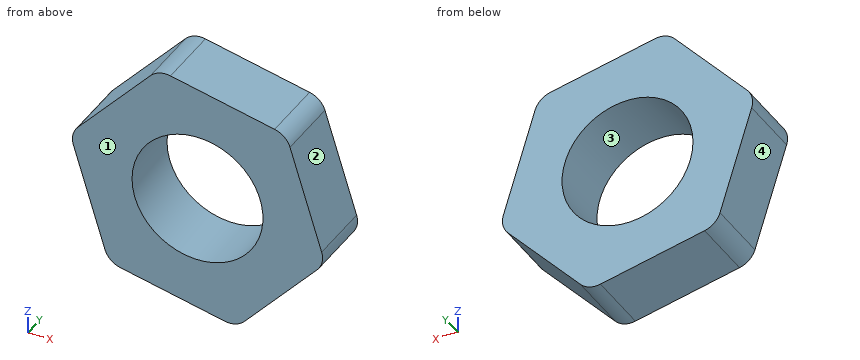
```python
from build123d import *

# Parameters (mm, degrees)
F1_DEPTH = 1.190625
F2_R     = 2.38125
F3_DEPTH = 2.38125
F4_R     = 0.762


with BuildPart() as f1:
    # F0 (on Front) → F1 (new body, symmetric)
    with BuildSketch(Plane.XZ):
        Polygon((-1.4126416008, 4.548169957), (-4.6451515239, 1.0507014657), (-3.2325099231, -3.4974684913), (1.4126416008, -4.548169957), (4.6451515239, -1.0507014657), (3.2325099231, 3.4974684913), align=None)
    extrude(amount=F1_DEPTH, both=True)

    # F2 (on face) → F3 (cut)
    with BuildSketch(Plane(origin=(0, 1.190625, 0), x_dir=(-1, 0, 0), z_dir=(0, 1, 0))):
        Circle(F2_R)
    extrude(amount=-F3_DEPTH, mode=Mode.SUBTRACT)

    # F4
    f4_edges = [f1.edges().sort_by_distance(p)[0] for p in [
        (-1.412642, 0, 4.54817),
        (3.23251, 0, 3.497468),
        (4.645152, 0, -1.050701),
        (1.412642, 0, -4.54817),
        (-3.23251, 0, -3.497468),
        (-4.645152, 0, 1.050701),
    ]]
    fillet(f4_edges, radius=F4_R)


solid = f1.part
```
CAD build for the part. Positions are in the model's coordinates, mm. Face numbers are marked on the shaded views. Round coordinates to 2 decimals unless told otherwise and drop trailing zeros. Write each loop counter-clockwise with the first axis right and the second up, starting at its lowest first coordinate (ties: lowest second). Pieces come first, ordered by that corner, then holes. Notation, with made-up numbers: (-10.5, 79) -> (12.5, 79) arc R5 ccw to (12.5, 83) -> close; hole circle Ø3 at (-20, 40.5). An arc over 180 degrees is marked (long way). Answer in a Markdown table with one row per item. Add a question column.
Item 1: Saw through at A-A, the plane y = 0.2. Write the cut outline in (x, z), then the cut area to 3 significant figures.
Item 2: Drill centre lines: line 1 (Z direction, x = 0, y = -0.25); line 2 (Z direction, x = 1.5, y = 0.15); line 3 (X direction, y = -1, z = 0.25). Where is each one in solid material? Low to high. Write a range as from..to.
Item 3: Saw through at C-C, the plane x = -0.5. Write the cut outline in (y, z).
Item 4: Mould opens along X. For the marked faces 1, 2, 3 and 4 say: pulls with the +X half, pulls with the -X half, needs draft (parallel to the pull), parting line crosses it, or undercut.
Item 5: Saw through at B-B, the plane z = 0. Write the cut outline in (x, y), then the cut area to 3 significant figures.
Item 6: Saw through at D-D, the plane x = 3.5. Write the cut outline in (y, z).
Item 7: Drop a flat-ended pin along its axis: pin 1 Ø1 at (x, y) = (0, -0.5) entering from +Z. Give the stop position or say it passes through.
Findings below:
| question | item | result |
|---|---|---|
| 1 | outline | (-4.51, 0.63) -> (-3.36, -3.08) arc R0.76 ccw to (-2.8, -3.59) -> (0.98, -4.45) arc R0.76 ccw to (1.71, -4.23) -> (4.35, -1.37) arc R0.76 ccw to (4.51, -0.63) -> (3.36, 3.08) arc R0.76 ccw to (2.8, 3.59) -> (-0.98, 4.45) arc R0.76 ccw to (-1.71, 4.23) -> (-4.35, 1.37) arc R0.76 ccw to start; hole circle Ø4.76 at (0, 0) |
| 1 | area | 40.9 mm^2 |
| 2 | line 1 | z = -4.23..-2.38, 2.38..4.23 |
| 2 | line 2 | z = -4.39..-1.85, 1.85..3.89 |
| 2 | line 3 | x = -4.4..-2.37, 2.37..4.24 |
| 3 | outline | (-1.19, -4.12) -> (1.19, -4.12) -> (1.19, -2.33) -> (-1.19, -2.33) -> close; (-1.19, 2.33) -> (1.19, 2.33) -> (1.19, 4.34) -> (-1.19, 4.34) -> close |
| 4 | face 1 | needs draft |
| 4 | face 2 | pulls with the +X half |
| 4 | face 3 | undercut |
| 4 | face 4 | pulls with the -X half |
| 5 | outline | (-4.32, -1.19) -> (-2.38, -1.19) -> (-2.38, 1.19) -> (-4.32, 1.19) -> close; (2.38, -1.19) -> (4.32, -1.19) -> (4.32, 1.19) -> (2.38, 1.19) -> close |
| 5 | area | 9.23 mm^2 |
| 6 | outline | (-1.19, -2.29) -> (1.19, -2.29) -> (1.19, 2.64) -> (-1.19, 2.64) -> close |
| 7 | pin 1 | stops at z = 4.34 |
